from build123d import *

# Parameters (mm, degrees)
SKETCH_1_R                       = 14.15
EXTRUDE_1_DEPTH                  = 26
SKETCH_2_R                       = 4
EXTRUDE_2_DEPTH                  = 14
CHAMFER1_SIZE                    = 0.8
HOLE_WIZARD_M3_1_D               = 2.5
HOLE_WIZARD_M3_1_DEPTH           = 8.5
HOLE_WIZARD_M3_1_TIP             = 0.751075774
CHAMFER_1_SIZE                   = 2.5
CHAMFER_1_SIZE2                  = 1
CUT_EXTRUDE_1_DEPTH              = 4
FILLET_1_R                       = 1
PATTERN_CIRCULAR_1_COUNT         = 5
FILLET_1_OF_PATTERN_CIRCULAR_1_R = 1
CHAMFER2_SIZE                    = 0.5
SKETCH2_W                        = 0.5
SKETCH2_H                        = 4.15
SKETCH2_W_2                      = 1
SKETCH2_H_2                      = 2.15
CHAMFER3_SIZE                    = 1
CHAMFER3_SIZE2                   = 2


# Read off the part's stored shape, not the designer's step: M6 Machine Threads Stud1
with BuildPart() as part:
    # 草图1 → 凸台-拉伸1 (new body)
    with BuildSketch(Plane(origin=(0, 0, 0), x_dir=(0, 0, -1), z_dir=(1, 0, 0))):
        with Locations(Location((0, 0, 0), (0, 0, 180))):
            Circle(SKETCH_1_R)
    extrude(amount=EXTRUDE_1_DEPTH)

    # 草图2 → 凸台-拉伸2 (add)
    with BuildSketch(Plane(origin=(26, 0, 0), x_dir=(0, 0, -1), z_dir=(1, 0, 0))):
        Circle(SKETCH_2_R)
    extrude(amount=EXTRUDE_2_DEPTH)

    # M6 Machine Threads Stud1 outline → M6 Machine Threads Stud1 (revolve, cut)
    with BuildSketch(Plane.YX):
        with BuildLine():
            Line((4, 40), (2.4585, 40))
            Line((2.4585, 40), (3, 39.4585))
            Line((3, 39.4585), (3, 35))
            Line((3, 35), (2.440192379, 34.030384758))
            ThreePointArc((2.440192379, 34.030384758), (2.410222252, 33.958030472), (2.4, 33.880384758))
            Line((2.4, 33.880384758), (2.4, 33.330384758))
            ThreePointArc((2.4, 33.330384758), (2.487867965, 33.118252723), (2.7, 33.030384758))
            Line((2.7, 33.030384758), (4, 33.030384758))
            Line((4, 33.030384758), (4, 40))
        make_face()
    revolve(axis=Axis((0, 0, 0), (1, 0, 0)), mode=Mode.SUBTRACT)

    # Chamfer1
    chamfer1_edges = [part.edges().sort_by_distance(p)[0] for p in [
        (33.030384758, 0, 4),
        (26, 0, 4),
    ]]
    chamfer(chamfer1_edges, length=CHAMFER1_SIZE)

    # M3 螺纹孔1
    with Locations(Plane.ZY):
        with Locations((8, 0), (0, 9.5), (0, -9.5), (-8, 0)):
            Hole(HOLE_WIZARD_M3_1_D / 2, depth=HOLE_WIZARD_M3_1_DEPTH)
            with Locations((0, 0, -(HOLE_WIZARD_M3_1_DEPTH + HOLE_WIZARD_M3_1_TIP / 2))):  # 118° drill point
                Cone(0, HOLE_WIZARD_M3_1_D / 2, HOLE_WIZARD_M3_1_TIP, mode=Mode.SUBTRACT)

    # 倒角1
    chamfer_1_edges = [part.edges().sort_by_distance(p)[0] for p in [
        (26, 0, -14.15),
    ]]
    chamfer_1_side = [part.faces().sort_by_distance(p)[0] for p in [
        (13, 0, -14.15),
    ]]
    chamfer(chamfer_1_edges, length=CHAMFER_1_SIZE, length2=CHAMFER_1_SIZE2, reference=chamfer_1_side[0])

    # 草图8 → 切除-拉伸1 (cut)
    with BuildSketch(Plane(origin=(26, 0, 0), x_dir=(0, 0, -1), z_dir=(1, 0, 0))):
        with BuildLine():
            Line((0, -5.238373922), (-5.676389324, -10.00143011))
            ThreePointArc((-5.676389324, -10.00143011), (0, -11.5), (5.676389324, -10.00143011))
            Line((5.676389324, -10.00143011), (0, -5.238373922))
        make_face()
    cut_extrude_1 = extrude(amount=-CUT_EXTRUDE_1_DEPTH, mode=Mode.SUBTRACT)

    # 圆角1
    fillet_1_edges = [part.edges().sort_by_distance(p)[0] for p in [
        (24, -10.00143011, 5.676389324),
        (24, -5.238373922, 0),
        (24, -10.00143011, -5.676389324),
    ]]
    fillet(fillet_1_edges, radius=FILLET_1_R)

    # 阵列(圆周)1: 切除-拉伸1 ×5 about axis
    pattern_circular_1_axis = Axis((0, 0, 0), (1, 0, 0))
    for i in range(1, PATTERN_CIRCULAR_1_COUNT):
        add(cut_extrude_1.rotate(pattern_circular_1_axis, i * 360 / PATTERN_CIRCULAR_1_COUNT), mode=Mode.SUBTRACT)

    # 圆角1 of 阵列(圆周)1
    fillet_1_of_pattern_circular_1_edges = [part.edges().sort_by_distance(p)[0] for p in [
        (24, -8.489178927, -7.757824511),
        (24, -1.618746565, -4.981989654),
        (24, 2.307955183, -11.266026046),
        (24, 4.754828997, -10.47098855),
        (24, 4.237933526, -3.079038938),
        (24, 11.427824858, -1.286397691),
        (24, 11.427824858, 1.286397691),
        (24, 4.237933526, 3.079038938),
        (24, 4.754828997, 10.47098855),
        (24, 2.307955183, 11.266026046),
        (24, -1.618746565, 4.981989654),
        (24, -8.489178927, 7.757824511),
    ]]
    fillet(fillet_1_of_pattern_circular_1_edges, radius=FILLET_1_OF_PATTERN_CIRCULAR_1_R)

    # Chamfer2
    chamfer2_edges = [part.edges().sort_by_distance(p)[0] for p in [
        (26, 0.155972278, 7.822133498),
        (26, -4.723918935, 6.236560727),
        (26, -3.553695435, 10.937149937),
        (26, -1.713122608, 5.272449246),
        (26, 1.526939092, 10.938601831),
        (26, -7.664868512, 7.952002496),
        (26, 7.487489119, 2.268833731),
        (26, 4.471550488, 6.419917137),
        (26, 9.303695435, 6.759530401),
        (26, 4.485013213, 3.258552838),
        (26, 10.875078679, 1.928008487),
        (26, 5.194229162, 9.747027055),
        (26, 4.471550488, -6.419917137),
        (26, 7.487489119, -2.268833731),
        (26, 9.303695435, -6.759530401),
        (26, 4.485013213, -3.258552838),
        (26, 5.194229162, -9.747027055),
        (26, 10.875078679, -1.928008487),
        (26, -4.723918935, -6.236560727),
        (26, 0.155972278, -7.822133498),
        (26, -3.553695435, -10.937149937),
        (26, -1.713122608, -5.272449246),
        (26, -7.664868512, -7.952002496),
        (26, 1.526939092, -10.938601831),
        (26, -7.39109295, 2.565510635),
        (26, -7.39109295, -2.565510635),
        (26, -11.5, 0),
        (26, -5.543781212, 0),
        (26, -9.931378421, 4.832419234),
        (26, -9.931378421, -4.832419234),
    ]]
    chamfer(chamfer2_edges, length=CHAMFER2_SIZE)

    # Sketch2 → Cut-Revolve1 (revolve, cut)
    with BuildSketch(Plane.XY, mode=Mode.PRIVATE) as cut_revolve1_sk:
        with Locations((7.25, 12.075)):
            Rectangle(SKETCH2_W, SKETCH2_H)
        with Locations((3.5, 13.075)):
            Rectangle(SKETCH2_W_2, SKETCH2_H_2)
        with Locations((5.5, 13.075)):
            Rectangle(SKETCH2_W_2, SKETCH2_H_2)
    revolve(cut_revolve1_sk.sketch.rotate(Axis((0, 0, 0), (1, 0, 0)), 90), axis=Axis((0, 0, 0), (1, 0, 0)), mode=Mode.SUBTRACT)

    # Chamfer3
    chamfer3_edges = [part.edges().sort_by_distance(p)[0] for p in [
        (0, 0, -14.15),
    ]]
    chamfer3_side = [part.faces().sort_by_distance(p)[0] for p in [
        (0, 0, 0),
    ]]
    chamfer(chamfer3_edges, length=CHAMFER3_SIZE, length2=CHAMFER3_SIZE2, reference=chamfer3_side[0])


solid = part.part
Read the model definition and answer for the solid it produces. Units are mm, in the model's axes. A direction names the side the tool comes from. Coordinates: 2 decimals unless noted, no trailing zeros. Loops run counter-clockwise (first coordinate to the right, second up) from the corner with the lowest first, then second, coordinate; pieces in that order, holes last. Notation, with made-up numbers: (-35.75, -17.75) -> (19.25, -17.75) arc R30 cw to (19.25, 7.25) -> close; hole circle Ø9 at (70, -27). An arc over 180 degrees is marked (long way). Answer in a Markdown table with one row per item.
Item 1: For faces 4 (the flat face through (23.77, 7.52, -2.26)), 5 (the flat face through (7.5, -10, -3)), 6 (the cylindrical face through (4.31, -8.26, 0.16)), determine the directions among +Z, -Z, +X, -X, +Y, -Y from which every point of the face is accessible in a straight line to the end or side of a thin tool.
Returned:
| item | result |
|---|---|
| face 4 | +X |
| face 5 | none |
| face 6 | -X |
Item 2: Straight lines are drawn through the part: line 1 along Y through (x, z) = (6.5, 0); line 2 along X through (y, z) = (-12.25, -2); line 3 along Y through (x, z) = (5.5, 0). For each, find the intervals that lie inside material, in ascending order. Write a range as [from, to].
Returned:
| item | result |
|---|---|
| line 1 | y = [-14.15, -10.75], [-8.25, 8.25], [10.75, 14.15] |
| line 2 | x = [0, 3], [4, 5], [6, 7], [7.5, 26] |
| line 3 | y = [-12, -10.75], [-8.25, 8.25], [10.75, 12] |
Item 3: A cutting plane is placed at C-C on x = 36. Determine the outline of the cut face in (y, z), plus the area to 3 significant figures.
Returned:
| item | result |
|---|---|
| outline | circle Ø6 at (0, 0) |
| area | 28.3 mm^2 |
Item 4: Each of these flat-tipped pins is pushed along its axis until it touches: P1, Ø3, axis at y = 9.5, z = 0, coming from the +X side; P2, Ø1, axis at x = 24, y = -6, coming from the -Z side; P3, Ø1.5, axis at y = 0, z = 8, coming from the -X side. Where does it stop, or does it pass through?
Returned:
| item | result |
|---|---|
| P1 | stops at x = 26 |
| P2 | stops at z = -12.91 |
| P3 | stops at x = 8.8 |
Item 5: A cutting plane is placed at B-B on x = 16.5. Determine the outline of the cut face in (y, z).
Returned:
| item | result |
|---|---|
| outline | circle Ø28.3 at (0, 0) |
Item 6: A cutting plane is placed at A-A on x = 23. Give the number of separate pieces and of enclosed holes in the cut face, plus the area to 3 significant figures.
Returned:
| item | result |
|---|---|
| separate pieces | 1 |
| enclosed holes | 5 |
| area | 443 mm^2 |
Item 7: For a pull along Y with two mould halves and no side action, classify faces 1 (the cylindrical face through (23.73, 1.53, 10.93)), 2 (the cylindrical face through (7.3, 0.2, 10)), 3 (the flat face through (7, -10, -3)) as released by +Y, released by -Y, zero draft, split by the parting line, or undercut.
Returned:
| item | result |
|---|---|
| face 1 | undercut |
| face 2 | split by the parting line |
| face 3 | zero draft |
